CAD build for the part. Positions are in the model's coordinates, mm. A direction names the side the tool comes from. Give positions to 0.01 mm unless a question says otherwise; leave off trailing zeros. Write each loop counter-clockwise with the first axis right and the second up, starting at its lowest first coordinate (ties: lowest second). Pieces come first, ordered by that corner, then holes. Notation, with made-up numbers: (42.25, -37.5) - (84.25, -37.5) arc R14 cw to (84.25, -19.5) - close; hole circle Ø5 at (53, 0). An arc over 180 degrees is marked (long way). Answer as a JSON object with one key per item and string values.
from build123d import *

# Parameters (mm, degrees)
SKETCH1_W           = 32
SKETCH1_H           = 32
BOSS_EXTRUDE1_DEPTH = 30
FILLET1_R           = 6
SKETCH2_R           = 0.8
CUT_EXTRUDE2_DEPTH  = 6


with BuildPart() as part:
    # Sketch1 → Boss-Extrude1 (new body)
    with BuildSketch(Plane(origin=(33.5, 0, 0), x_dir=(0, 0, -1), z_dir=(1, 0, 0))):
        Rectangle(SKETCH1_W, SKETCH1_H)
    extrude(amount=BOSS_EXTRUDE1_DEPTH)

    # Fillet1
    fillet1_edges = [part.edges().sort_by_distance(p)[0] for p in [
        (63.5, 0, -16),
        (63.5, 16, 0),
        (63.5, 0, 16),
        (33.5, 16, 0),
        (33.5, 0, -16),
        (33.5, -16, 0),
        (33.5, 0, 16),
        (48.5, 16, 16),
        (48.5, 16, -16),
        (48.5, -16, -16),
        (48.5, -16, 16),
        (63.5, -16, 0),
    ]]
    fillet(fillet1_edges, radius=FILLET1_R)

    # Sketch2 → Cut-Extrude2 (cut)
    with BuildSketch(Plane(origin=(33.5, 0, 0), x_dir=(0, 0, -1), z_dir=(1, 0, 0))):
        with Locations((-4.5, -4.5)):
            Circle(SKETCH2_R)
        with Locations((4.5, -4.5)):
            Circle(SKETCH2_R)
        with Locations((-4.5, 4.5)):
            Circle(SKETCH2_R)
        with Locations((4.5, 4.5)):
            Circle(SKETCH2_R)
    extrude(amount=CUT_EXTRUDE2_DEPTH, mode=Mode.SUBTRACT)


solid = part.part
(1) Pull direction Z, two halves, no side cores. Call faces 1 (the face through (48.626, 14.196, -14.289)), 2 (the face through (39.5, 4.5, 4.5)), 3 (the face through (61.696, -14.289, -0.14)): pulls with the +Z half, pulls with the -Z half, needs draft (parallel to the pull), parting line crosses it, or undercut.
Answer key:
{"face 1": "pulls with the -Z half", "face 2": "undercut", "face 3": "needs draft"}
(2) Flat gauge pin, fed straight in: P1, Ø1.3, axis at y = 4.5, z = 4.5, coming from the -X side. Where does the tip first touch, or does it go through?
Answer key:
{"P1": "stops at x = 39.5"}
(3) Probe L1, parallel to Y at x = 36.65, z = -4.5; L2, parallel to Y at x = 35.65, z = 4.5; L3, parallel to Y at x = 39.5, z = 11. List the from-to ranges inside material, lowest first. Write a range as [from, to].
Answer key:
{"L1": "y = [-15.28, -5.3], [-3.7, 3.7], [5.3, 15.28]", "L2": "y = [-14.6, -5.3], [-3.7, 3.7], [5.3, 14.6]", "L3": "y = [-15.92, 15.92]"}
(4) Saw through at D-D, the plane x = 38.25. Give the cut face in (y, z), and give its area (3 significant figures).
Answer key:
{"outline": "(-15.87, -10) arc R5.87 ccw to (-10, -15.87) - (10, -15.87) arc R5.87 ccw to (15.87, -10) - (15.87, 10) arc R5.87 ccw to (10, 15.87) - (-10, 15.87) arc R5.87 ccw to (-15.87, 10) - close; hole circle Ø1.6 at (-4.5, -4.5); hole circle Ø1.6 at (-4.5, 4.5); hole circle Ø1.6 at (4.5, -4.5); hole circle Ø1.6 at (4.5, 4.5)", "area": "970 mm²"}
(5) Saw through at A-A, the plane y = 4.5. Give the cut face in (x, z).
Answer key:
{"outline": "(33.5, -10) arc R6 ccw to (39.5, -16) - (57.5, -16) arc R6 ccw to (63.5, -10) - (63.5, 10) arc R6 ccw to (57.5, 16) - (39.5, 16) arc R6 ccw to (33.5, 10) - (33.5, 5.3) - (39.5, 5.3) - (39.5, 3.7) - (33.5, 3.7) - (33.5, -3.7) - (39.5, -3.7) - (39.5, -5.3) - (33.5, -5.3) - close"}
(6) 3-axis set-ups, long thin cutter, end or side, ignore diameter. For faces 4 (the face through (48, -16, 0)), 5 (the face through (39.5, 4.5, -4.5)): which of +Z, -Z, +X, -X, +Y, -Y reach the whole face in a straight line?
Answer key:
{"face 4": "+Z, -Z, +X, -X, -Y", "face 5": "-X"}
(7) Saw through at B-B, the plane x = 54. Give the cut face in (y, z), and give its area (3 significant figures).
Answer key:
{"outline": "(-16, -10) arc R6 ccw to (-10, -16) - (10, -16) arc R6 ccw to (16, -10) - (16, 10) arc R6 ccw to (10, 16) - (-10, 16) arc R6 ccw to (-16, 10) - close", "area": "993 mm²"}
